from build123d import *

# Parameters (mm, degrees)
SKETCH1_W                   = 100
SKETCH1_H                   = 100
BOSS_EXTRUDE1_DEPTH         = 300
FILLET1_R                   = 10
SKETCH5_W                   = 80
SKETCH5_H                   = 60
SKETCH5_R                   = 10
BOSS_EXTRUDE2_DEPTH         = 10
FILLET2_RADIUS              = 40
FILLET2_LENGTH              = 10
FILLET2_OF_MIRROR1_2_RADIUS = 40
FILLET2_OF_MIRROR1_2_LENGTH = 10


with BuildPart() as part:
    # Sketch1 → Boss-Extrude1 (new body)
    with BuildSketch(Plane(origin=(0, 0, 0), x_dir=(1, 0, 0), z_dir=(0, 1, 0))):
        Rectangle(SKETCH1_W, SKETCH1_H)
    extrude(amount=BOSS_EXTRUDE1_DEPTH)

    # Fillet1
    fillet1_edges = [part.edges().sort_by_distance(p)[0] for p in [
        (50, 150, 50),
        (-50, 150, 50),
        (-50, 150, -50),
        (50, 150, -50),
    ]]
    fillet(fillet1_edges, radius=FILLET1_R)

    # Sketch5 → Boss-Extrude2 (add)
    with BuildSketch(Plane(origin=(50, 0, 0), x_dir=(0, 0, -1), z_dir=(1, 0, 0))):
        with Locations((0, 330)):
            Rectangle(SKETCH5_W, SKETCH5_H)
        with Locations((0, 340)):
            Circle(SKETCH5_R, mode=Mode.SUBTRACT)
    boss_extrude2 = extrude(amount=-BOSS_EXTRUDE2_DEPTH)

    # Fillet2: full round fillet: the end face becomes a half cylinder, R = half its width
    fillet2_face = Plane((45, 360, 0), x_dir=(-1, 0, 0), z_dir=(0, 1, 0))  # on the end face: x along it, z out of the body
    fillet2_slab = fillet2_face.offset(-FILLET2_RADIUS / 2) * Box(FILLET2_LENGTH, 2 * FILLET2_RADIUS, FILLET2_RADIUS, mode=Mode.PRIVATE)  # the body's end, R deep
    fillet2_round = Plane((45, 320, 0), x_dir=(0, 1, 0), z_dir=(-1, 0, 0)) * Cylinder(FILLET2_RADIUS, FILLET2_LENGTH, mode=Mode.PRIVATE)  # its axis R under the face
    add(fillet2_slab - fillet2_round, mode=Mode.SUBTRACT)

    # Mirror1: Boss-Extrude2 across plane
    add(boss_extrude2.mirror(Plane(origin=(0, 0, 0), x_dir=(0, 0, 1), z_dir=(1, 0, 0))))

    # Fillet2 of Mirror1 2: full round fillet: the end face becomes a half cylinder, R = half its width
    fillet2_of_mirror1_2_face = Plane((-45, 360, 0), x_dir=(1, 0, 0), z_dir=(0, 1, 0))  # on the end face: x along it, z out of the body
    fillet2_of_mirror1_2_slab = fillet2_of_mirror1_2_face.offset(-FILLET2_OF_MIRROR1_2_RADIUS / 2) * Box(FILLET2_OF_MIRROR1_2_LENGTH, 2 * FILLET2_OF_MIRROR1_2_RADIUS, FILLET2_OF_MIRROR1_2_RADIUS, mode=Mode.PRIVATE)  # the body's end, R deep
    fillet2_of_mirror1_2_round = Plane((-45, 320, 0), x_dir=(0, 1, 0), z_dir=(1, 0, 0)) * Cylinder(FILLET2_OF_MIRROR1_2_RADIUS, FILLET2_OF_MIRROR1_2_LENGTH, mode=Mode.PRIVATE)  # its axis R under the face
    add(fillet2_of_mirror1_2_slab - fillet2_of_mirror1_2_round, mode=Mode.SUBTRACT)


solid = part.part
Read the model definition and answer for the solid it produces. Units are mm, in the model's axes. A direction names the side the tool comes from. Give positions to 0.01 mm unless a question says otherwise; leave off trailing zeros. Write each loop counter-clockwise with the first axis right and the second up, starting at its lowest first coordinate (ties: lowest second). Pieces come first, ordered by that corner, then holes. Notation, with made-up numbers: (13, 41) - (21, 41) arc R27 cw to (21, 58) - close; hole circle Ø1 at (12.5, 41.25). An arc over 180 degrees is marked (long way). Use CSV: the item, a comma, the result in double quotes. Start each with the question number.
Item 1: For faces 4 (the flat face through (-1, 148, 50)), 5 (the flat face through (-45, 310, 40)), 6 (the flat face through (45, 310, -40)), 7 (the flat face through (50, 183, 1)), 8 (the flat face through (40, 324, 1)), determine the directions among +Z, -Z, +X, -X, +Y, -Y from which every point of the face is accessible in a straight line to the end or side of a thin tool.
Item 2: The part is cut by section A-A, the plane z = 0. Give the vertices of the cut face in (x, y), and give its area (3 significant figures).
Item 3: The mould has two halves that part along Y. Classify faces 1 (the cylindrical face through (-44.93, 359.99, -0.88)), 2 (the cylindrical face through (45.07, 349.915, 1.302)), 3 (the cylindrical face through (46.99, 152.1, 47.15)): pulls with the +Y half, pulls with the -Y half, needs draft (parallel to the pull), parting line crosses it, or undercut.
Item 4: Consider line 1 (Y direction, x = 47.5, z = 0); line 2 (X direction, y = 344, z = 21); line 3 (Y direction, x = -16.5, z = -0.5). Determine where each line is inside the solid, lowest interval first.
Item 5: The part is cut by section D-D, the plane z = -30. Give the vertices of the cut face in (x, y), and give its area (3 significant figures).
Item 6: Flat-ended cylindrical pins translate along their axes: P1, Ø5, axis at x = 47, y = 305.5, coming from the +Z side; P2, Ø5, axis at x = 46, y = 310, coming from the -Z side; P3, Ø8, axis at x = 18, z = 37.5, coming from the +Y side. Find the tip coordinate at first contact, or state that the pin passes through.
Item 7: The part is cut by section C-C, the plane x = 29. Give the vertices of the cut face in (y, z).
Item 8: The part is cut by section B-B, the plane y = 340. Give the vertices of the cut face in (x, z), and give its area (3 significant figures).
Taken from the geometry:
1,face 4,"+Z, +X, -X, +Y, -Y"
1,face 5,"+Z, +X, -X, +Y"
1,face 6,"-Z, +X, -X, +Y"
1,face 7,"+Z, -Z, +X, +Y, -Y"
1,face 8,"+Z, -Z, +Y"
2,outline,"(-50, 0) - (50, 0) - (50, 330) - (40, 330) - (40, 300) - (-40, 300) - (-40, 330) - (-50, 330) - close; (-50, 350) - (-40, 350) - (-40, 360) - (-50, 360) - close; (40, 350) - (50, 350) - (50, 360) - (40, 360) - close"
2,area,"30,800 mm2"
3,face 1,"pulls with the +Y half"
3,face 2,"undercut"
3,face 3,"needs draft"
4,line 1,"0 to 330, 350 to 360"
4,line 2,"-50 to -40, 40 to 50"
4,line 3,"0 to 300"
5,outline,"(-50, 0) - (50, 0) - (50, 346.46) - (40, 346.46) - (40, 300) - (-40, 300) - (-40, 346.46) - (-50, 346.46) - close"
5,area,"30,900 mm2"
6,P1,"z = 40"
6,P2,"z = -40"
6,P3,"y = 300"
7,outline,"(0, -50) - (300, -50) - (300, 50) - (0, 50) - close"
8,outline,"(-50, -34.64) - (-40, -34.64) - (-40, -10) - (-50, -10) - close; (-50, 10) - (-40, 10) - (-40, 34.64) - (-50, 34.64) - close; (40, -34.64) - (50, -34.64) - (50, -10) - (40, -10) - close; (40, 10) - (50, 10) - (50, 34.64) - (40, 34.64) - close"
8,area,"986 mm2"
